Could you check a few things on this model? Use its own coordinates, in mm. Face numbers are marked on the shaded views. Coordinates: 2 decimals unless noted, no trailing zeros. Order: outer loops, then holes, each group sorted by start corner. A loop starts at its lowest first (then second) coordinate and runs counter-clockwise, first axis right, second up. Notation, with made-up numbers: (48.5, 6) -> (67.5, 6) arc R19 cw to (67.5, 34) -> close; hole circle Ø4 at (68.25, 3). An arc over 180 degrees is marked (long way). Use a Markdown table: item, result. Add a question column.
1) If we section it at D-D (y = 33): Write out the boundary of the cut face in (x, z).
2) If I drill on L1, parallel to Z at x = 34, y = 17; L2, parallel to Y at x = 0, z = 7.5; L3, parallel to Y at x = -4, z = 5, over which ranges is the centre line in solid material (lowest first)? Write a range as [from, to].
3) Thinking about a two-plate mould opening in X: for the marked faces 1, 2 and 3, which applies, +X half, -X half, draft (parallel to the pull), parting line (faces both ways), or undercut?
4) Will these pins go through, and if not, where does the flat tip stop? pin 1 Ø1 at (y, z) = (2.5, 8.5) entering from +X; pin 2 Ø4 at (y, z) = (19, 1.5) entering from -X; pin 3 Ø6 at (y, z) = (27, 10.5) entering from +X.
5) If we section it at A-A (x = 0): Write out the boundary of the cut face in (y, z), plus the area to 3 significant figures.
6) If we section it at C-C (z = 5.75): Write out the boundary of the cut face in (x, y).
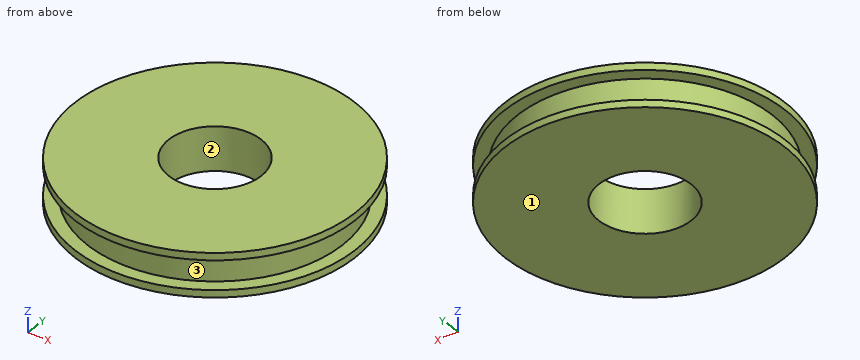
```python
from build123d import *

# Parameters (mm, degrees)
F0_R     = 38.5
F0_R_2   = 35
F0_R_3   = 12.7
F1_DEPTH = 2
F2_DEPTH = 10
F3_R     = 38.5
F3_R_2   = 35
F3_R_3   = 12.7
F4_DEPTH = 2


with BuildPart() as f1:
    # F0 (on Top) → F1 (new body)
    with BuildSketch(Plane.XY):
        Circle(F0_R)
        Circle(F0_R_2, mode=Mode.SUBTRACT)
        Circle(F0_R_2)
        Circle(F0_R_3, mode=Mode.SUBTRACT)
    extrude(amount=F1_DEPTH)

    # F0 (on Top) → F2 (join)
    with BuildSketch(Plane.XY):
        Circle(F0_R_2)
        Circle(F0_R_3, mode=Mode.SUBTRACT)
    extrude(amount=F2_DEPTH)

    # F3 (on face) → F4 (join)
    with BuildSketch(Plane.XY.offset(10)):
        Circle(F3_R)
        Circle(F3_R_2, mode=Mode.SUBTRACT)
        Circle(F3_R_2)
        Circle(F3_R_3, mode=Mode.SUBTRACT)
    extrude(amount=F4_DEPTH)


solid = f1.part
```
Answer sheet:
| question | item | result |
|---|---|---|
| 1 | outline | (-19.83, 0) -> (19.83, 0) -> (19.83, 2) -> (11.66, 2) -> (11.66, 10) -> (19.83, 10) -> (19.83, 12) -> (-19.83, 12) -> (-19.83, 10) -> (-11.66, 10) -> (-11.66, 2) -> (-19.83, 2) -> close |
| 2 | L1 | [0, 2], [10, 12] |
| 2 | L2 | [-35, -12.7], [12.7, 35] |
| 2 | L3 | [-34.77, -12.05], [12.05, 34.77] |
| 3 | face 1 | draft |
| 3 | face 2 | undercut |
| 3 | face 3 | parting line |
| 4 | pin 1 | x = 34.94 |
| 4 | pin 2 | x = -34.54 |
| 4 | pin 3 | x = 30.1 |
| 5 | outline | (-38.5, 0) -> (-12.7, 0) -> (-12.7, 12) -> (-38.5, 12) -> (-38.5, 10) -> (-35, 10) -> (-35, 2) -> (-38.5, 2) -> close; (12.7, 0) -> (38.5, 0) -> (38.5, 2) -> (35, 2) -> (35, 10) -> (38.5, 10) -> (38.5, 12) -> (12.7, 12) -> close |
| 5 | area | 563 mm2 |
| 6 | outline | circle Ø70 at (0, 0); hole circle Ø25.4 at (0, 0) |
